from build123d import *

# Parameters (mm, degrees)
EXTRUDE_1_DEPTH        = 32
SKETCH_2_R             = 1.5
EXTRUDE_2_DEPTH        = 6
HOLE_WIZARD_M3_1_D     = 2.5
HOLE_WIZARD_M3_1_DEPTH = 3.9
HOLE_WIZARD_M3_1_TIP   = 0.751075774


with BuildPart() as part:
    # 草图1 → 凸台-拉伸1 (new body)
    with BuildSketch(Plane.XY):
        Polygon((4.041451884, 0), (2.020725942, 3.5), (-2.020725942, 3.5), (-4.041451884, 0), (-2.020725942, -3.5), (2.020725942, -3.5), align=None)
    extrude(amount=EXTRUDE_1_DEPTH)

    # 草图2 → 凸台-拉伸2 (add)
    with BuildSketch(Plane.XY.offset(32)):
        Circle(SKETCH_2_R)
    extrude(amount=EXTRUDE_2_DEPTH)

    # M3 螺纹孔1
    with Locations(Plane(origin=(0, 0, 0), x_dir=(-1, 0, 0), z_dir=(0, 0, -1))):
        with Locations((0, 0)):
            Hole(HOLE_WIZARD_M3_1_D / 2, depth=HOLE_WIZARD_M3_1_DEPTH)
            with Locations((0, 0, -(HOLE_WIZARD_M3_1_DEPTH + HOLE_WIZARD_M3_1_TIP / 2))):  # 118° drill point
                Cone(0, HOLE_WIZARD_M3_1_D / 2, HOLE_WIZARD_M3_1_TIP, mode=Mode.SUBTRACT)


solid = part.part
Part model, mm, in its own coordinate system. A direction names the side the tool comes from. Give positions to 0.01 mm unless a question says otherwise; leave off trailing zeros. Write each loop counter-clockwise with the first axis right and the second up, starting at its lowest first coordinate (ties: lowest second). Pieces come first, ordered by that corner, then holes.
1) Cut at C-C on y = -2.5. Write the cut outline in (x, z).
Resolved:
outline: (-2.6, 0) - (2.6, 0) - (2.6, 32) - (-2.6, 32) - close
2) Cut at A-A on z = 7. Write the cut outline in (x, y).
Resolved:
outline: (-4.04, 0) - (-2.02, -3.5) - (2.02, -3.5) - (4.04, 0) - (2.02, 3.5) - (-2.02, 3.5) - close
3) Two-plate mould, pull along X, no slides. Class faces 4 (the face through (-1.5, 0.07, 34.96)), 5 (the face through (-3.045, -1.726, 15.776)), 6 (the face through (0.05, -0.21, 4.52)): released by +X, released by -X, zero draft, split by the parting line, or undercut.
Resolved:
face 4: split by the parting line
face 5: released by -X
face 6: undercut
4) Cut at B-B on x = -2.75. Write the cut outline in (y, z).
Resolved:
outline: (-2.24, 0) - (2.24, 0) - (2.24, 32) - (-2.24, 32) - close
5) Pin check, flat tips, straight feed: pin 1 (4 mm diameter, centred on x = 0, y = 0, fed in from -Z); pin 2 (1 mm diameter, centred on x = -3, y = 1, fed in from +Z). Stop position of each tip, or through.
Resolved:
pin 1: stops at z = 0
pin 2: stops at z = 32
6) Which spindle directions (+Z, -Z, +X, -X, +Y, -Y) get a long thin tool onto all of the face, cutting with end or side? Do faces 1 (the face through (2, 0, 32)), 2 (the face through (0, -3.5, 16)), 3 (the face through (-0.27, -1.22, 1.98)). Say none if no direction does.
Resolved:
face 1: +Z
face 2: +Z, -Z, +X, -X, -Y
face 3: -Z
7) Probe L1, parallel to Y at x = 0, z = 2.3; L2, parallel to Z at x = -1.5, y = 0.75; L3, parallel to X at y = 0.25, z = 3. List the from-to ranges inside material, lowest first.
Resolved:
L1: y = -3.5 to -1.25, 1.25 to 3.5
L2: z = 0 to 32
L3: x = -3.9 to -1.22, 1.22 to 3.9
